The listing builds one solid part. Answer for the finished solid, in the listing's coordinates (mm). A direction names the side the tool comes from. Give positions to 0.01 mm unless a question says otherwise; leave off trailing zeros. Order: outer loops, then holes, each group sorted by start corner. A loop starts at its lowest first (then second) coordinate and runs counter-clockwise, first axis right, second up. Notation, with made-up numbers: (74, 13.5) - (89, 13.5) arc R25 ccw to (89, 48.5) - close; hole circle Ø8 at (27, -29.75). An arc over 180 degrees is marked (long way). Use CSV: the item, a comma, the result in double quotes.
```python
from build123d import *

# Parameters (mm, degrees)
SKETCH1_W           = 12.1
SKETCH1_H           = 22.5
BOSS_EXTRUDE1_DEPTH = 22.5
BOSS_EXTRUDE2_DEPTH = 4.5
SKETCH2_3_R         = 2.5
BOSS_EXTRUDE3_DEPTH = 7.2
SKETCH9_R           = 1.27
BOSS_EXTRUDE7_DEPTH = 3
SKETCH12_W          = 12.175
SKETCH12_H          = 5
SKETCH12_W_2        = 12.1
BOSS_EXTRUDE8_DEPTH = 19.8
SKETCH12_2_W        = 12.175
SKETCH12_2_H        = 5
SKETCH12_2_W_2      = 12.1
CUT_EXTRUDE1_DEPTH  = 17.3


with BuildPart() as part:
    # Sketch1 → Boss-Extrude1 (new body)
    with BuildSketch(Plane(origin=(0, 0, 0), x_dir=(1, 0, 0), z_dir=(0, 1, 0))):
        Rectangle(SKETCH1_W, SKETCH1_H)
    extrude(amount=BOSS_EXTRUDE1_DEPTH)

    # Sketch2 → Boss-Extrude2 (add)
    with BuildSketch(Plane(origin=(0, 22.5, 0), x_dir=(1, 0, 0), z_dir=(0, 1, 0))):
        with BuildLine():
            ThreePointArc((-2.445144707, 0.229166667), (0, -11.25), (2.445144707, 0.229166667))
            ThreePointArc((2.445144707, 0.229166667), (0, 3.25), (-2.445144707, 0.229166667))
        make_face()
    extrude(amount=BOSS_EXTRUDE2_DEPTH)

    # Sketch2<3> → Boss-Extrude3 (add)
    with BuildSketch(Plane(origin=(0, 22.5, 0), x_dir=(1, 0, 0), z_dir=(0, 1, 0))):
        with Locations((0, -5.25)):
            Circle(SKETCH2_3_R)
    extrude(amount=BOSS_EXTRUDE3_DEPTH)

    # Sketch9 → Boss-Extrude7 (add)
    with BuildSketch(Plane.XY.offset(11.25)):
        with Locations((0, 1.27)):
            Circle(SKETCH9_R)
        with Locations((-2.6, 1.27)):
            Circle(SKETCH9_R)
        with Locations((2.6, 1.27)):
            Circle(SKETCH9_R)
    extrude(amount=BOSS_EXTRUDE7_DEPTH)

    # Sketch12 → Boss-Extrude8 (add)
    with BuildSketch(Plane.XZ):
        with Locations((0.0375, 13.75)):
            Rectangle(SKETCH12_W, SKETCH12_H)
        with Locations((0, -13.75)):
            Rectangle(SKETCH12_W_2, SKETCH12_H)
    extrude(amount=-BOSS_EXTRUDE8_DEPTH)

    # Sketch12<2> → Cut-Extrude1 (cut)
    with BuildSketch(Plane.XZ):
        with Locations((0.0375, 13.75)):
            Rectangle(SKETCH12_2_W, SKETCH12_2_H)
        with Locations((0, -13.75)):
            Rectangle(SKETCH12_2_W_2, SKETCH12_2_H)
    extrude(amount=-CUT_EXTRUDE1_DEPTH, mode=Mode.SUBTRACT)


solid = part.part
```
Item 1: The part is cut by section D-D (z = 5.25). Give the vertices of the cut face in (x, y), and give its area (3 significant figures).
Taken from the geometry:
outline,"(-6.05, 0) - (6.05, 0) - (6.05, 22.5) - (6, 22.5) - (6, 27) - (2.5, 27) - (2.5, 29.7) - (-2.5, 29.7) - (-2.5, 27) - (-6, 27) - (-6, 22.5) - (-6.05, 22.5) - close"
area,"340 mm^2"
Item 2: Each of these flat-tipped pins is pushed along its axis until it touches: pin 1 (4 mm diameter, centred on x = -1, y = 13, fed in from +Z); pin 2 (0.8 mm diameter, centred on x = -0.5, y = 21.5, fed in from -Z); pin 3 (7 mm diameter, centred on y = 15.5, z = -4.5, fed in from +X). Where does it stop, or does it pass through?
Taken from the geometry:
pin 1,"z = 11.25"
pin 2,"z = -11.25"
pin 3,"x = 6.05"
Item 3: Find the intervals of material crossed by line 1 along Z through (x, y) = (-5.25, 6.5); line 2 along Y through (x, z) = (-3, -8); line 3 along X through (y, z) = (6.75, -0.5), in increasing order.
Taken from the geometry:
line 1,"-11.25 to 11.25"
line 2,"0 to 22.5"
line 3,"-6.05 to 6.05"
Item 4: The mould has two halves that part along Y. Classify faces 1 (the face through (0, 17.3, -14)), 2 (the face through (0, 19.8, -14)), 3 (the face through (0, 19, -16.25)): +Y half, -Y half, draft (parallel to the pull), parting line (faces both ways), or undercut.
Taken from the geometry:
face 1,"-Y half"
face 2,"+Y half"
face 3,"draft"
Item 5: The part is cut by section C-C (y = 20.5). Give the vertices of the cut face in (x, z).
Taken from the geometry:
outline,"(-6.05, -11.25) - (6.05, -11.25) - (6.05, 11.25) - (-6.05, 11.25) - close"
Item 6: Which of the six approach directions +Z, -Z, +X, -X, +Y, -Y give full straight-line access (tool end or side, diameter ignored) to faces 4 (the face through (0, 21, 11.25)), 5 (the face through (0, 21, -11.25)), 6 (the face through (0, 9, -11.25)), 7 (the face through (-0.33, 28.33, 2.77))?
Taken from the geometry:
face 4,"+Z, +X, -X, +Y"
face 5,"-Z, +X, -X, +Y"
face 6,"-Z, +X, -X, -Y"
face 7,"+Y"
Item 7: The part is cut by section A-A (z = -0.75). Give the vertices of the cut face in (x, y), and give its area (3 significant figures).
Taken from the geometry:
outline,"(-6.05, 0) - (6.05, 0) - (6.05, 22.5) - (2.5, 22.5) - (2.5, 27) - (-2.5, 27) - (-2.5, 22.5) - (-6.05, 22.5) - close"
area,"295 mm^2"
